Part print with two shaded views. Sizes in mm from the minimum x, y, z corner. A direction names the side the tool comes from. Round coordinates to 2 decimals unless told otherwise and drop trailing zeros. Loops run counter-clockwise (first coordinate to the right, second up) from the corner with the lowest first, then second, coordinate; pieces in that order, holes last. Notation, with made-up numbers: M 85.5,24 L 141.5,24 A25 cw 141.5,46 Z; hole C 38.5,35.25 d7. An arc over 180 degrees is marked long. Put each result on its own line as item: value. Start each with the question number.
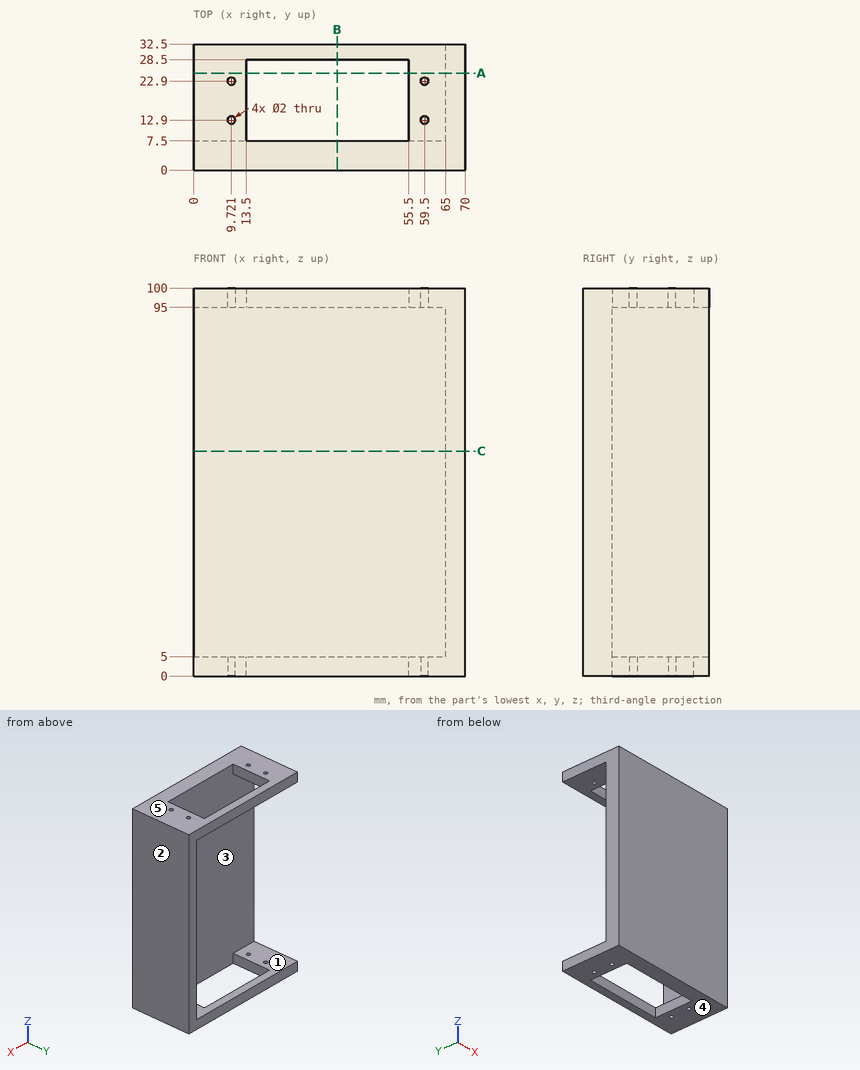
(1) Tool access for the marked faces 1 and 2: list every direction of +Z, -Z, +X, -X, +Y, -Y with a clear straight run to the whole face (end or side of a thin tool).
(2) Cut at A-A on y = 25. List the corners of the cut face in (x, z).
(3) Cut at C-C on z = 58. List the corners of the cut face in (x, y), and give its area (3 significant figures).
(4) Mould opens along Z. For the marked faces 3, 4 and 5 say: +Z half, -Z half, draft (parallel to the pull), parting line (faces both ways), or undercut.
(5) Flat gauge pins, fed straight in: pin 1 Ø3 at (x, y) = (9.72, 22.9) entering from -Z; pin 2 Ø2 at (y, z) = (16, 83.5) entering from -X; pin 3 Ø1 at (x, y) = (54.5, 18) entering from +Z. Where does each tip first touch, or does it go through?
(6) Drill centre lines: line 1 along Y through (x, z) = (59.5, 2.15); line 2 along X through (y, z) = (22.9, 3.45); line 3 along X through (y, z) = (12, 98) (1 decimal). Where is each one in solid material? Low to high.
(7) Cut at B-B on x = 37. List the corners of the cut face in (y, z), and give its area (3 significant figures).
Taken from the geometry:
1. face 1: -X, +Y
1. face 2: +Z, -Z, +X, +Y, -Y
2. outline: M 0,0 L 13.5,0 L 13.5,5 L 0,5 Z; M 0,95 L 13.5,95 L 13.5,100 L 0,100 Z; M 55.5,0 L 70,0 L 70,100 L 55.5,100 L 55.5,95 L 65,95 L 65,5 L 55.5,5 Z
3. outline: M 0,0 L 70,0 L 70,32.5 L 65,32.5 L 65,7.5 L 0,7.5 Z
3. area: 650 mm2
4. face 3: undercut
4. face 4: -Z half
4. face 5: +Z half
5. pin 1: z = 0
5. pin 2: x = 65
5. pin 3: through
6. line 1: 0 to 11.9, 13.9 to 21.9, 23.9 to 32.5
6. line 2: 0 to 8.72, 10.72 to 13.5, 55.5 to 58.5, 60.5 to 70
6. line 3: 0 to 9.3, 10.2 to 13.5, 55.5 to 59.1, 59.9 to 70
7. outline: M 0,0 L 7.5,0 L 7.5,100 L 0,100 Z; M 28.5,0 L 32.5,0 L 32.5,5 L 28.5,5 Z; M 28.5,95 L 32.5,95 L 32.5,100 L 28.5,100 Z
7. area: 790 mm2
